```python
from build123d import *

# Parameters (mm, degrees)
SKETCH1_W                                        = 30
SKETCH1_H                                        = 57
BOSS_EXTRUDE1_DEPTH                              = 3.9
SKETCH2_R                                        = 5
CUT_EXTRUDE1_DEPTH                               = 65.530690373
F_4_0_4_DIAMETER_HOLE1_D                         = 4
SKETCH12_W                                       = 14.5
SKETCH12_H                                       = 24
CUT_EXTRUDE2_DEPTH                               = 65.530690373
CBORE_FOR_M3_PAN_HEAD_MACHINE_SCREW2_D           = 3.2
CBORE_FOR_M3_PAN_HEAD_MACHINE_SCREW2_CBORE_D     = 9
CBORE_FOR_M3_PAN_HEAD_MACHINE_SCREW2_CBORE_DEPTH = 1
CSK_FOR_M3_FLAT_HEAD_MACHINE_SCREW1_D            = 3.2
CSK_FOR_M3_FLAT_HEAD_MACHINE_SCREW1_CSINK_D      = 4
CSK_FOR_M3_FLAT_HEAD_MACHINE_SCREW1_CSINK_ANGLE  = 90
SKETCH19_W                                       = 4
SKETCH19_H                                       = 33
CUT_EXTRUDE3_DEPTH                               = 65.530690373


with BuildPart() as part:
    # Sketch1 → Boss-Extrude1 (new body)
    with BuildSketch(Plane(origin=(0, 0, 0), x_dir=(0, 0, -1), z_dir=(1, 0, 0))):
        with Locations((-15, 28.5)):
            Rectangle(SKETCH1_W, SKETCH1_H)
    extrude(amount=-BOSS_EXTRUDE1_DEPTH)

    # Sketch2 → Cut-Extrude1 (cut, through all)
    with BuildSketch(Plane(origin=(0, 0, 0), x_dir=(0, 0, -1), z_dir=(1, 0, 0))):
        with Locations((-7, 23.5)):
            Circle(SKETCH2_R)
    extrude(amount=-CUT_EXTRUDE1_DEPTH, mode=Mode.SUBTRACT)

    # Ø4.0 (4) Diameter Hole1 (through all)
    with Locations(Plane(origin=(0, 4.5, 7), x_dir=(0, 0, 1), z_dir=(1, 0, 0))):
        with Locations((0, 0)):
            Hole(F_4_0_4_DIAMETER_HOLE1_D / 2)

    # Sketch12 → Cut-Extrude2 (cut, through all)
    with BuildSketch(Plane(origin=(0, 0, 0), x_dir=(0, 0, -1), z_dir=(1, 0, 0))):
        with Locations((-22.75, 12)):
            Rectangle(SKETCH12_W, SKETCH12_H)
    extrude(amount=-CUT_EXTRUDE2_DEPTH, mode=Mode.SUBTRACT)

    # CBORE for M3 Pan Head Machine Screw2 (through all)
    with Locations(Plane(origin=(-3.9, 41.360571099, 16), x_dir=(0, 0, -1), z_dir=(-1, 0, 0))):
        with Locations((0, 0)):
            CounterBoreHole(CBORE_FOR_M3_PAN_HEAD_MACHINE_SCREW2_D / 2, CBORE_FOR_M3_PAN_HEAD_MACHINE_SCREW2_CBORE_D / 2, CBORE_FOR_M3_PAN_HEAD_MACHINE_SCREW2_CBORE_DEPTH)

    # CSK for M3 Flat Head Machine Screw1 (through all)
    with Locations(Plane(origin=(0, 30.032608687, 19.33966579), x_dir=(0, 0, 1), z_dir=(1, 0, 0))):
        with Locations((0, 0), (-14.431341448, -7.272)):
            CounterSinkHole(CSK_FOR_M3_FLAT_HEAD_MACHINE_SCREW1_D / 2, CSK_FOR_M3_FLAT_HEAD_MACHINE_SCREW1_CSINK_D / 2, counter_sink_angle=CSK_FOR_M3_FLAT_HEAD_MACHINE_SCREW1_CSINK_ANGLE)

    # Sketch19 → Cut-Extrude3 (cut, through all)
    with BuildSketch(Plane.ZY.offset(3.9)):
        with Locations((28, 40.5)):
            Rectangle(SKETCH19_W, SKETCH19_H)
    extrude(amount=-CUT_EXTRUDE3_DEPTH, mode=Mode.SUBTRACT)


solid = part.part
```
Read the model definition and answer for the solid it produces. Units are mm, in the model's axes. A direction names the side the tool comes from. Give positions to 0.01 mm unless a question says otherwise; leave off trailing zeros. Order: outer loops, then holes, each group sorted by start corner. A loop starts at its lowest first (then second) coordinate and runs counter-clockwise, first axis right, second up.
(1) Find section A-A (y = 4.5). Give the vertices of the cut face in (x, z).
(2) Find section D-D (z = 22). Give the vertices of the cut face in (x, y), plus the area to 3 significant figures.
(3) Straight lines are drawn through the part: L1, parallel to Y at x = -1.5, z = 16; L2, parallel to Y at x = -1.55, z = 4; L3, parallel to Y at x = -3.7, z = 8.5. For each, find the intervals that lie inside material, in ascending order.
(4) Find section B-B (x = -1.1). Give the vertices of the cut face in (y, z), plus the area to 3 significant figures.
(5) For a pull along Y with two mould halves and no side action, classify faces 4 (the flat face through (-2, 40, 26)), 5 (the flat face through (-2, 0, 8)), 6 (the cylindrical face through (-1.43, 42.92, 15.65)) as released by +Y, released by -Y, zero draft, split by the parting line, or undercut.
(6) Find section C-C (y = 20.5). Give the vertices of the cut face in (x, z), plus the area to 4 significant figures.
(7) Given pin 1 (2.5 mm diameter, centred on y = 37.3, z = 4.91, fed in from +X); pin 2 (7 mm diameter, centred on y = 42, z = 16, fed in from -X); pin 3 (1.2 mm diameter, centred on x = -2.5, z = 21.5, fed in from -Y); pin 4 (1.2 mm diameter, centred on x = -1.5, y = 10, fed in from +Z), each flat-ended and moving along its own axis, determine where each tip first touches the part or whether it passes through.
(8) For faces 1 (the flat face through (-2, 24, 21)), 2 (the flat face through (-2, 28, 0)), 3 (the cylindrical face through (-3.407, 45.754, 16.976)), determine the directions among +Z, -Z, +X, -X, +Y, -Y from which every point of the face is accessible in a straight line to the end or side of a thin tool.
Result sheet:
1. outline: (-3.9, 0) - (0, 0) - (0, 5) - (-3.9, 5) - close; (-3.9, 9) - (0, 9) - (0, 15.5) - (-3.9, 15.5) - close
2. outline: (-3.9, 24) - (0, 24) - (0, 57) - (-3.9, 57) - close
2. area: 129 mm2
3. L1: y = 24 to 39.76, 42.96 to 57
3. L2: y = 0 to 19.5, 27.5 to 35.99, 38.62 to 57
3. L3: y = 0 to 3.18, 5.82 to 18.73, 28.27 to 57
4. outline: (0, 0) - (57, 0) - (57, 26) - (24, 26) - (24, 15.5) - (0, 15.5) - close; hole circle Ø4 at (4.5, 7); hole circle Ø10 at (23.5, 7); hole circle Ø3.2 at (30.03, 19.34); hole circle Ø3.2 at (37.3, 4.91); hole circle Ø3.2 at (41.36, 16)
4. area: 1,110 mm2
5. face 4: zero draft
5. face 5: released by -Y
5. face 6: undercut
6. outline: (-3.9, 0) - (0, 0) - (0, 3) - (-3.9, 3) - close; (-3.9, 11) - (0, 11) - (0, 15.5) - (-3.9, 15.5) - close
6. area: 29.25 mm2
7. pin 1: passes through
7. pin 2: stops at x = -2.9
7. pin 3: stops at y = 24
7. pin 4: stops at z = 15.5
8. face 1: +Z, +X, -X, -Y
8. face 2: -Z, +X, -X, +Y, -Y
8. face 3: -X
